Answer from the drawing. Dimensions are ordinates in mm from the lowest x, y and z of the part. Give positions to 0.01 mm unless a question says otherwise; leave off trailing zeros. Order: outer loops, then holes, each group sorted by start corner. A loop starts at its lowest first (then second) coordinate and runs counter-clockwise, first axis right, second up. Notation, with made-up numbers: (27.5, 66.5) -> (44.5, 66.5) arc R7 ccw to (44.5, 71.5) -> close; hole circle Ø1 at (-17, 40). An arc over 180 degrees is marked (long way). One line per question, with ' | ' between items. Start each with the question number.
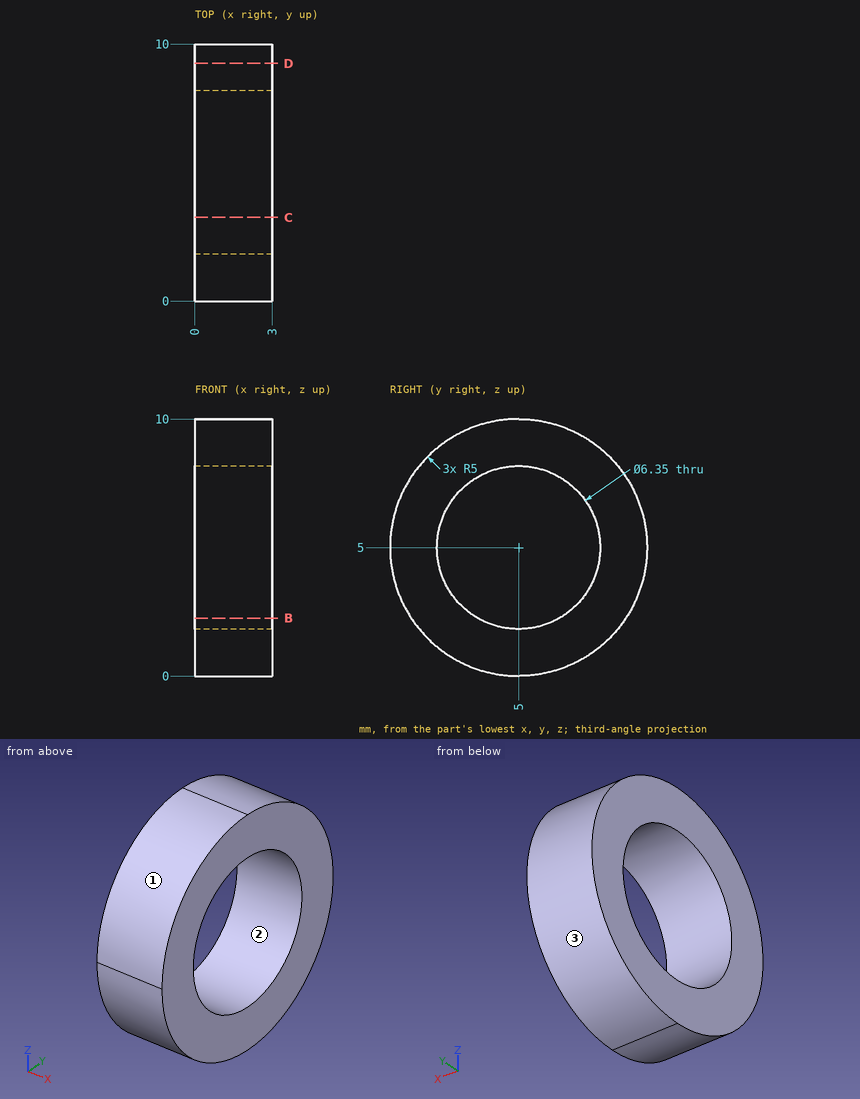
(1) The part is cut by section B-B on z = 2.25. Determine the outline of the cut face in (x, y), plus the area to 3 significant figures.
(2) The part is cut by section D-D on y = 9.25. Determine the outline of the cut face in (x, z), plus the area to 3 significant figures.
(3) Determine the mould class of the marked faces 1, 2 and 3 for opening direction Z: pulls with the +Z half, pulls with the -Z half, needs draft (parallel to the pull), parting line crosses it, or undercut.
(4) The part is cut by section C-C on y = 3.25. Determine the outline of the cut face in (x, z), plus the area to 3 significant figures.
(5) Given P1, Ø1, axis at x = 2, y = 1.5, coming from the +Z side; P2, Ø1.5, axis at x = 1.5, z = 4, coming from the -Y side; P3, Ø1.5, axis at x = 2.5, z = 1.5, coming from the -Y side, each flat-ended and moving along its own axis, determine where each tip first touches the part or whether it passes through.
(6) Consider line 1 (Y direction, x = 1.7, z = 5) (3 decimals); line 2 (Z direction, x = 1.2, y = 7.25) (1 decimal); line 3 (Z direction, x = 2.1, y = 6.25). Determine where each line is inside the solid, lowest interval first.
Result sheet:
1) outline: (0, 0.82) -> (3, 0.82) -> (3, 3.41) -> (0, 3.41) -> close; (0, 6.59) -> (3, 6.59) -> (3, 9.18) -> (0, 9.18) -> close | area: 15.5 mm^2
2) outline: (0, 2.37) -> (3, 2.37) -> (3, 7.63) -> (0, 7.63) -> close | area: 15.8 mm^2
3) face 1: pulls with the +Z half | face 2: undercut | face 3: parting line crosses it
4) outline: (0, 0.32) -> (3, 0.32) -> (3, 2.35) -> (0, 2.35) -> close; (0, 7.65) -> (3, 7.65) -> (3, 9.68) -> (0, 9.68) -> close | area: 12.2 mm^2
5) P1: stops at z = 9 | P2: stops at y = 0.01 | P3: stops at y = 0.82
6) line 1: y = 0 to 1.825, 8.175 to 10 | line 2: z = 0.5 to 2.8, 7.2 to 9.5 | line 3: z = 0.16 to 2.08, 7.92 to 9.84
